Geometry: final body of the model. Coordinates: model frame, mm. Give positions to 0.01 mm unless a question says otherwise; leave off trailing zeros. Order: outer loops, then holes, each group sorted by start corner. A loop starts at its lowest first (then second) coordinate and runs counter-clockwise, first axis right, second up. Notation, with made-up numbers: (13, 7.25) -> (33, 7.25) arc R18 cw to (33, 23.25) -> close; hole circle Ø9 at (22, -14.75). An arc over 180 degrees is marked (long way). One line per question, with ' | ' between items. Start each with the question number.
(1) Section C-C (x = 0.6). Return loops of the section in (y, z).
(2) Section B-B (y = 0). Return loops of the section in (x, z), then the cut area to 3 significant figures.
(3) First-contact query: pin 1 Ø2.5 at (y, z) = (7, -5) entering from -X. Flat tip, straight axial feed; report the tip coordinate or a pass-through.
(4) Section D-D (z = 4). Return loops of the section in (x, y).
(5) Section A-A (z = -5). Return loops of the section in (x, y).
(6) Ray query, L1, parallel to Y at x = 2.8, z = -5; L2, parallel to Y at x = 2, z = -56; L3, parallel to Z at x = 0.25, y = -2.25. Return the intervals inside material, ascending.
```python
from build123d import *

# Parameters (mm, degrees)
SKETCH_1_R      = 8.5
SKETCH_1_R_2    = 1.5
EXTRUDE_1_DEPTH = 4


with BuildPart() as part:
    # 草图1 → 凸台-拉伸1 (new body)
    with BuildSketch(Plane(origin=(0, 0, 0), x_dir=(0, 0, -1), z_dir=(1, 0, 0))):
        with BuildLine():
            Line((-9, 12), (0, 12))
            Line((0, 12), (56, 12))
            ThreePointArc((56, 12), (68, 0), (56, -12))
            Line((56, -12), (0, -12))
            Line((0, -12), (-9, -12))
            ThreePointArc((-9, -12), (-21, 0), (-9, 12))
        make_face()
        with Locations((56, 0)):
            Circle(SKETCH_1_R, mode=Mode.SUBTRACT)
        with Locations((5, 7)):
            Circle(SKETCH_1_R_2, mode=Mode.SUBTRACT)
        with Locations((5, -7)):
            Circle(SKETCH_1_R_2, mode=Mode.SUBTRACT)
        with Locations((-9, 0)):
            Circle(SKETCH_1_R, mode=Mode.SUBTRACT)
    extrude(amount=EXTRUDE_1_DEPTH)


solid = part.part
```
Response:
1) outline: (-12, -56) arc R12 ccw to (12, -56) -> (12, 9) arc R12 ccw to (-12, 9) -> close; hole circle Ø17 at (0, -56); hole circle Ø3 at (-7, -5); hole circle Ø17 at (0, 9); hole circle Ø3 at (7, -5)
2) outline: (0, -68) -> (4, -68) -> (4, -64.5) -> (0, -64.5) -> close; (0, -47.5) -> (4, -47.5) -> (4, 0.5) -> (0, 0.5) -> close; (0, 17.5) -> (4, 17.5) -> (4, 21) -> (0, 21) -> close | area: 220 mm^2
3) pin 1: passes through
4) outline: (0, -12) -> (4, -12) -> (4, -6.87) -> (0, -6.87) -> close; (0, 6.87) -> (4, 6.87) -> (4, 12) -> (0, 12) -> close
5) outline: (0, -12) -> (4, -12) -> (4, -8.5) -> (0, -8.5) -> close; (0, -5.5) -> (4, -5.5) -> (4, 5.5) -> (0, 5.5) -> close; (0, 8.5) -> (4, 8.5) -> (4, 12) -> (0, 12) -> close
6) L1: y = -12 to -8.5, -5.5 to 5.5, 8.5 to 12 | L2: y = -12 to -8.5, 8.5 to 12 | L3: z = -67.79 to -64.2, -47.8 to 0.8, 17.2 to 20.79
